from build123d import *

# Parameters (mm, degrees)
F1_DEPTH        = 10
F2_DEPTH        = 10
F2_COPIES_COUNT = 7
F4_R            = 12.2091154471
F5_DEPTH        = 5


# Not quite as in the source:
# - a pattern or mirror of a feature is missing from the dataset's text; its kind, count and spacing are read off the source's solid


with BuildPart() as f1:
    # F0 (on Top) → F1 (new body)
    with BuildSketch(Plane.XY):
        with BuildLine():
            ThreePointArc((4.3237516011, -6.4317705254), (6.8400137028, -3.6437223475), (7.75, 0))
            ThreePointArc((7.75, 0), (6.5755629687, 4.1017644551), (3.4082008658, 6.9603639889))
            ThreePointArc((3.4082008658, 6.9603639889), (1.7433706712, 7.5513680021), (-0.0120479028, 7.7499906354))
            ThreePointArc((-0.0120479028, 7.7499906354), (-5.6679911875, 5.2854872905), (-7.7319524669, -0.5285934635))
            ThreePointArc((-7.7319524669, -0.5285934635), (-3.4082008658, -6.9603639889), (4.3237516011, -6.4317705254))
        make_face()
        with BuildLine():
            ThreePointArc((-2, -1.5), (-2.5, 0), (-2, 1.5))
            Line((-2, 1.5), (2, 1.5))
            ThreePointArc((2, 1.5), (2.5, 0), (2, -1.5))
            Line((2, -1.5), (-2, -1.5))
        make_face(mode=Mode.SUBTRACT)
    extrude(amount=F1_DEPTH)

    # F0 (on Top) → F2 (join)
    with BuildSketch(Plane.XY):
        with BuildLine():
            ThreePointArc((-0.0120479028, 7.7499906354), (1.7433706712, 7.5513680021), (3.4082008658, 6.9603639889))
            Line((3.4082008658, 6.9603639889), (4.3726173887, 8.9377108908))
            add(Edge.make_bspline(
                [(4.3726173887, 8.9377108908), (4.3837213667, 9.6011226956), (4.2995730436, 10.8287649694), (3.902399388, 11.5686550219)],
                knots=[0, 0, 0, 0, 2.6726339048, 2.6726339048, 2.6726339048, 2.6726339048], degree=3))
            Line((3.902399388, 11.5686550219), (1.5639112325, 12.1085375524))
            add(Edge.make_bspline(
                [(-0.0120479028, 9.9499906354), (0.2687925016, 10.5511288793), (0.8825874647, 11.6176382491), (1.5639112325, 12.1085375524)],
                knots=[0, 0, 0, 0, 2.6726339048, 2.6726339048, 2.6726339048, 2.6726339048], degree=3))
            Line((-0.0120479028, 9.9499906354), (-0.0120479028, 7.7499906354))
        make_face()
    f2 = extrude(amount=F2_DEPTH)

    # F2_copies: F2 ×7 about axis
    f2_copies_axis = Axis((0, 0, 0), (0, 0, 1))
    for i in range(1, F2_COPIES_COUNT):
        add(f2.rotate(f2_copies_axis, i * 360 / F2_COPIES_COUNT))

    # F4 (on face) + F0 (on Top) → F5 (join)
    with BuildSketch(Plane.XY):
        Circle(F4_R)
        with BuildLine():
            ThreePointArc((7.75, 0), (6.8400137028, -3.6437223475), (4.3237516011, -6.4317705254))
            ThreePointArc((4.3237516011, -6.4317705254), (-3.4082008658, -6.9603639889), (-7.7319524669, -0.5285934635))
            ThreePointArc((-7.7319524669, -0.5285934635), (-5.6679911875, 5.2854872905), (-0.0120479028, 7.7499906354))
            ThreePointArc((-0.0120479028, 7.7499906354), (1.7433706712, 7.5513680021), (3.4082008658, 6.9603639889))
            ThreePointArc((3.4082008658, 6.9603639889), (6.5755629687, 4.1017644551), (7.75, 0))
        make_face(mode=Mode.SUBTRACT)
    with BuildSketch(Plane.XY):
        with BuildLine():
            ThreePointArc((4.3237516011, -6.4317705254), (6.8400137028, -3.6437223475), (7.75, 0))
            ThreePointArc((7.75, 0), (6.5755629687, 4.1017644551), (3.4082008658, 6.9603639889))
            ThreePointArc((3.4082008658, 6.9603639889), (1.7433706712, 7.5513680021), (-0.0120479028, 7.7499906354))
            ThreePointArc((-0.0120479028, 7.7499906354), (-5.6679911875, 5.2854872905), (-7.7319524669, -0.5285934635))
            ThreePointArc((-7.7319524669, -0.5285934635), (-3.4082008658, -6.9603639889), (4.3237516011, -6.4317705254))
        make_face()
        with BuildLine():
            ThreePointArc((-2, -1.5), (-2.5, 0), (-2, 1.5))
            Line((-2, 1.5), (2, 1.5))
            ThreePointArc((2, 1.5), (2.5, 0), (2, -1.5))
            Line((2, -1.5), (-2, -1.5))
        make_face(mode=Mode.SUBTRACT)
    extrude(amount=-F5_DEPTH)


solid = f1.part
Can you work these out from the model? Positions are in its coordinate system, mm. A direction names the side the tool comes from. Coordinates: 2 decimals unless noted, no trailing zeros. Write each loop counter-clockwise with the first axis right and the second up, starting at its lowest first coordinate (ties: lowest second). Pieces come first, ordered by that corner, then holes. Notation, with made-up numbers: (-38.5, 41) - (-18.5, 41) arc R17 ccw to (-18.5, 49) - close; hole circle Ø5 at (5.25, 0.5). An arc over 180 degrees is marked (long way). Return JSON: item names as keys, results as strings. Group by question number.
Item 1: Which directions (+Z, -Z, +X, -X, +Y, -Y) give clear straight access to the entire face, cutting with the end or side of a thin tool? Please do faces 1 (the face through (2.658, -11.856, 4.93)), 2 (the face through (6.924, 5.537, 4.93)), 3 (the face through (-2.5, 0, 2.6)), 4 (the face through (10.967, 5.229, 4.93)).
Item 2: I'm going to push flat-ended pins straight in: pin 1 Ø6 at (y, z) = (5.5, 0.5) entering from +X; pin 2 Ø1 at (y, z) = (3, 3) entering from -X; pin 3 Ø1 at (y, z) = (-0.5, 2.5) entering from +X. Where does each tip first touch, or does it pass through?
Item 3: We'd pull the mould along X, two halves only. Please class faces 5 (the face through (-6.94, 5.52, 4.93)), 6 (the face through (0, -1.5, 3)), 7 (the face through (0, -3, -5)): pulls with the +X half, pulls with the -X half, needs draft (parallel to the pull), parting line crosses it, or undercut.
Item 4: Please list where these lines run through material, in increasing order: probe 1 along Y at (x, z) = (1, 3.25); probe 2 along Z at (x, y) = (8, 7.5); probe 3 along X at (y, z) = (9.5, 9).
Item 5: If we section it at C-C (x = -9): Write out the boundary of the cut face in (y, z), then the cut area to 3 significant figures.
Item 6: If we section it at A-A (z = -3.75): Write out the boundary of the cut face in (x, y).
Item 7: If we section it at B-B (y = 5.75): Write out the boundary of the cut face in (x, z).
Return value:
{
 "1": {"face 1": "+Z, +X, -Y", "face 2": "+Z, +Y", "face 3": "+Z, -Z", "face 4": "+Z, +X, +Y"},
 "2": {"pin 1": "stops at x = 11.94", "pin 2": "stops at x = -7.34", "pin 3": "stops at x = 7.75"},
 "3": {"face 5": "pulls with the -X half", "face 6": "undercut", "face 7": "needs draft"},
 "4": {"probe 1": "y = -11.64 to -1.5, 1.5 to 11.57", "probe 2": "z = -5 to 0", "probe 3": "x = -7.57 to -4.95, -0.01 to 4.36"},
 "5": {"outline": "(-8.25, -5) - (8.25, -5) - (8.25, 0) - (2.11, 0) - (2.11, 10) - (-2.07, 10) - (-2.07, 0) - (-8.25, 0) - close", "area": "124 mm^2"},
 "6": {"outline": "circle Ø24.42 at (0, 0); hole (-2, -1.5) - (2, -1.5) arc R2.5 ccw to (2, 1.5) - (-2, 1.5) arc R2.5 ccw to start"},
 "7": {"outline": "(-10.77, -5) - (10.77, -5) - (10.77, 0) - (10.72, 0) - (10.72, 10) - (7.19, 10) - (7.19, 0) - (5.2, 0) - (5.2, 10) - (-7.23, 10) - (-7.23, 0) - (-10.77, 0) - close"}
}
